Read the model definition and answer for the solid it produces. Units are mm, in the model's axes. Face numbers are marked on the shaded views. Give positions to 0.01 mm unless a question says otherwise; leave off trailing zeros. Loops run counter-clockwise (first coordinate to the right, second up) from the corner with the lowest first, then second, coordinate; pieces in that order, holes last.
(1) Straight lines are drawn through the part: probe 1 along Y at (x, z) = (10, 0.5); probe 2 along Y at (x, z) = (0, 8); probe 3 along X at (y, z) = (-0.5, 11). For each, find the intervals that lie inside material, in ascending order.
(2) Find section B-B, the plane y = -35. Write down the section's boundary in (x, z), then the cut area to 3 significant figures.
(3) Find section C-C, the plane x = -37. Write down the section's boundary in (y, z).
(4) This flat-tipped pin is pushed along its axis until it touches: P1, Ø2.5, axis at x = -10, y = -16.5, coming from the +Z side. Where does it stop, or does it pass through?
(5) Determine the mould class of the marked faces 1, 2 and 3 for opening direction X: pulls with the +X half, pulls with the -X half, needs draft (parallel to the pull), parting line crosses it, or undercut.
(6) Find section A-A, the plane x = -5. Write down the section's boundary in (y, z) (3 decimals), then the cut area to 3 significant figures.
```python
from build123d import *

# Parameters (mm, degrees)
SKETCH_1_R          = 45
EXTRUDE_1_DEPTH     = 1
SKETCH_2_R          = 1
CUT_EXTRUDE_1_DEPTH = 64.647466564
SKETCH_3_R          = 13.5
SKETCH_3_R_2        = 12.2
EXTRUDE_2_DEPTH     = 6
SKETCH_4_R          = 4
CUT_EXTRUDE_2_DEPTH = 64.921827258
SKETCH_5_R          = 8
CUT_EXTRUDE_3_DEPTH = 10
SKETCH_6_R          = 13.5
SKETCH_6_R_2        = 12.2
EXTRUDE_3_DEPTH     = 8
SKETCH_7_R          = 0.4
CUT_EXTRUDE_4_DEPTH = 2.8


with BuildPart() as part:
    # 草图1 → 凸台-拉伸1 (new body)
    with BuildSketch(Plane.XY):
        Circle(SKETCH_1_R)
    extrude(amount=EXTRUDE_1_DEPTH)

    # 草图2 → 切除-拉伸1 (cut, through all)
    with BuildSketch(Plane.XY.offset(1)):
        with Locations((20, -16.5)):
            Circle(SKETCH_2_R)
        with Locations((20, 16.5)):
            Circle(SKETCH_2_R)
        with Locations((-20, 16.5)):
            Circle(SKETCH_2_R)
        with Locations((-20, -16.5)):
            Circle(SKETCH_2_R)
        with Locations((10, -16.5)):
            Circle(SKETCH_2_R)
        with Locations((10, 16.5)):
            Circle(SKETCH_2_R)
        with Locations((-10, 16.5)):
            Circle(SKETCH_2_R)
        with Locations((-10, -16.5)):
            Circle(SKETCH_2_R)
    extrude(amount=-CUT_EXTRUDE_1_DEPTH, mode=Mode.SUBTRACT)

    # 草图3 → 凸台-拉伸2 (add)
    with BuildSketch(Plane.XY.offset(1)):
        Circle(SKETCH_3_R)
        Circle(SKETCH_3_R_2, mode=Mode.SUBTRACT)
    extrude(amount=EXTRUDE_2_DEPTH)

    # 草图4 → 切除-拉伸2 (cut, through all)
    with BuildSketch(Plane.XY.offset(1)):
        Circle(SKETCH_4_R)
    extrude(amount=-CUT_EXTRUDE_2_DEPTH, mode=Mode.SUBTRACT)

    # 草图5 → 切除-拉伸3 (cut)
    with BuildSketch(Plane.XY.offset(1)):
        Circle(SKETCH_5_R)
    extrude(amount=-CUT_EXTRUDE_3_DEPTH, mode=Mode.SUBTRACT)

    # 草图6 → 凸台-拉伸3 (add)
    with BuildSketch(Plane.XY.offset(7)):
        Circle(SKETCH_6_R)
        Circle(SKETCH_6_R_2, mode=Mode.SUBTRACT)
    extrude(amount=EXTRUDE_3_DEPTH)

    # 草图7 → 切除-拉伸4 (cut)
    with BuildSketch(Plane(origin=(65.728441972, -2.343791879, 15), x_dir=(0.9999857974272592, -0.005329628858411386, 0), z_dir=(0, 0, 1))):
        with Locations(Location((-64.698660153, 14.801186776, 0), (0, 0, 0.305366686))):
            Circle(SKETCH_7_R)
        with Locations(Location((-66.781339847, -10.814285995, 0), (0, 0, 0.305366686))):
            Circle(SKETCH_7_R)
    extrude(amount=-CUT_EXTRUDE_4_DEPTH, mode=Mode.SUBTRACT)


solid = part.part
```
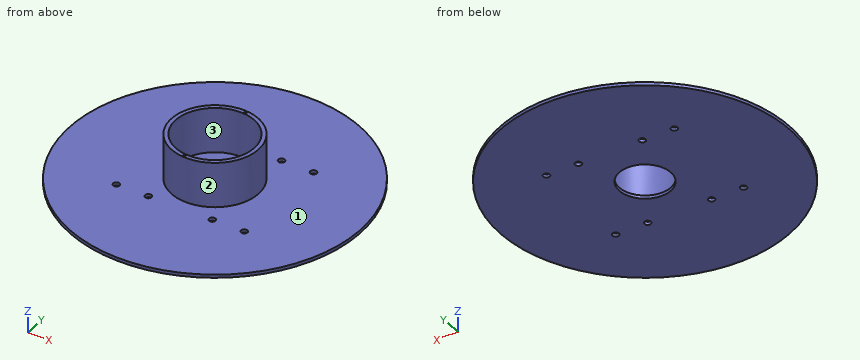
Entries:
1. probe 1: y = -43.87 to -17.5, -15.5 to 15.5, 17.5 to 43.87
1. probe 2: y = -13.5 to -12.2, 12.2 to 13.5
1. probe 3: x = -13.49 to -12.19, 12.19 to 13.49
2. outline: (-28.28, 0) - (28.28, 0) - (28.28, 1) - (-28.28, 1) - close
2. area: 56.6 mm2
3. outline: (-25.61, 0) - (25.61, 0) - (25.61, 1) - (-25.61, 1) - close
4. P1: stops at z = 1
5. face 1: needs draft
5. face 2: parting line crosses it
5. face 3: undercut
6. outline: (-44.721, 0) - (-6.245, 0) - (-6.245, 1) - (-11.128, 1) - (-11.128, 15) - (-12.54, 15) - (-12.54, 1) - (-44.721, 1) - close; (6.245, 0) - (44.721, 0) - (44.721, 1) - (12.54, 1) - (12.54, 15) - (11.128, 15) - (11.128, 1) - (6.245, 1) - close
6. area: 116 mm2
